Source: CAD feature listing. Evaluate the final solid. Frame: model axes, mm. A direction names the side the tool comes from. Coordinates: 2 decimals unless noted, no trailing zeros. Loops run counter-clockwise (first coordinate to the right, second up) from the corner with the lowest first, then second, coordinate; pieces in that order, holes last. Notation, with made-up numbers: (-1, 0.5) - (30, 0.5) arc R10 cw to (30, 6.5) - close; hole circle Ø8 at (62, -23.75). An arc over 180 degrees is marked (long way). Write item = value, one per line. Start each with the question number.
from build123d import *

# Parameters (mm, degrees)
F3_D     = 6.5278
F3_DEPTH = 28.575
F3_TIP   = 1.9611489744
F5_D     = 6.5278
F5_DEPTH = 28.575
F5_TIP   = 1.9611489744
F6_SIZE  = 0.635


with BuildPart() as f1:
    # F0 (on Front) → F1 (revolve)
    with BuildSketch(Plane.XZ):
        with BuildLine():
            Line((-95.25, 0), (0, 0))
            Line((0, 0), (0, 12.7))
            Line((0, 12.7), (-6.35, 12.7))
            ThreePointArc((-6.35, 12.7), (-8.674261314, 10.375738686), (-11.849261314, 9.525))
            Line((-11.849261314, 9.525), (-83.400738686, 9.525))
            ThreePointArc((-83.400738686, 9.525), (-86.575738686, 10.375738686), (-88.9, 12.7))
            Line((-88.9, 12.7), (-95.25, 12.7))
            Line((-95.25, 12.7), (-95.25, 0))
        make_face()
    revolve(axis=Axis((-50.5691878498, 0, 0), (-1, 0, 0)))

    # F3
    with Locations(Plane.YZ):
        with Locations((0, 0)):
            Hole(F3_D / 2, depth=F3_DEPTH)
            with Locations((0, 0, -(F3_DEPTH + F3_TIP / 2))):  # 118° drill point
                Cone(0, F3_D / 2, F3_TIP, mode=Mode.SUBTRACT)

    # F5
    with Locations(Plane(origin=(-95.25, 0, 0), x_dir=(0, -1, 0), z_dir=(-1, 0, 0))):
        with Locations((0, 0)):
            Hole(F5_D / 2, depth=F5_DEPTH)
            with Locations((0, 0, -(F5_DEPTH + F5_TIP / 2))):  # 118° drill point
                Cone(0, F5_D / 2, F5_TIP, mode=Mode.SUBTRACT)

    # F6
    f6_edges = [f1.edges().sort_by_distance(p)[0] for p in [
        (0, 0, -12.7),
        (-95.25, 0, -12.7),
    ]]
    chamfer(f6_edges, length=F6_SIZE)


solid = f1.part
Item 1: Draft query along Z for faces 4 (the cylindrical face through (-3.53, -12.4, -2.75)), 5 (the conical face through (-65.05, 0.12, -0.55)), 6 (the flat face through (-95.25, -3, 3)). Return one class per face: released by +Z, released by -Z, zero draft, split by the parting line, or undercut.
Item 2: Cut plane B-B (x = -51). Return the cut outline in (y, z) (3 decimals).
Item 3: First-contact query: pin 1 (12 mm diameter, centred on x = -18.5, y = 3.5, fed in from -Z) (3 decimals); pin 2 (5 mm diameter, centred on y = 0, z = 0, fed in from +X); pin 3 (6 mm diameter, centred on x = -64, z = 9, fed in from -Y); pin 4 (2 mm diameter, centred on y = 6, z = 0, fed in from +X). Flat tips, straight axial feed; report the tip coordinate or a pass-through.
Item 4: Reachability of faces 1 (the cylindrical face through (-14.488, 0.708, -3.186)), 2 (the cylindrical face through (-80.762, -0.708, -3.186)), 3 (the cylindrical face through (-48.126, -5.796, -7.559)) from +Z, -Z, +X, -X, +Y, -Y: full face, straight path, thin tool, end or side. Return the list, or none.
Item 5: Cut plane A-A (x = -14). Return the cut outline in (y, z) (3 decimals).
Item 6: Material intervals for L1, parallel to Y at x = -21, z = 0 (3 decimals); L2, parallel to Y at x = -6, z = 0; L3, parallel to Z at x = -22, y = -1, sorted ascending. Write a range as [from, to].
Responses:
q1.face_4 = split by the parting line
q1.face_5 = undercut
q1.face_6 = zero draft
q2.outline = circle Ø19.05 at (0, 0)
q3.pin_1 = -9.525
q3.pin_2 = -29.03
q3.pin_3 = -7.4
q3.pin_4 = 0
q4.face_1 = +X
q4.face_2 = -X
q4.face_3 = none
q5.outline = circle Ø19.05 at (0, 0); hole circle Ø6.528 at (0, 0)
q6.L1 = [-9.525, -3.264], [3.264, 9.525]
q6.L2 = [-12.7, -3.26], [3.26, 12.7]
q6.L3 = [-9.47, -3.11], [3.11, 9.47]
